Design review of the part built by this model. Coordinates are the model's own, in mm. A direction names the side the tool comes from. Coordinates: 2 decimals unless noted, no trailing zeros. Write each loop counter-clockwise with the first axis right and the second up, starting at its lowest first coordinate (ties: lowest second). Pieces come first, ordered by that corner, then holes.
Q1. Clearance check with flat-ended pins moving along their axes: pin 1 Ø1.5 at (x, y) = (6, 11) entering from +Z; pin 2 Ø1 at (x, y) = (9, -10.5) entering from -Z; pin 3 Ø10 at (x, y) = (6.5, 12) entering from +Z. State where each tip first meets the part, or that it passes through.
Q2. Add section D-D, the plane y = -15.5. Give the boundary of the cut face in (x, z), plus the area to 3 significant figures.
Q3. Add section A-A, the plane z = 0. Give the boundary of the cut face in (x, y), plus the area to 3 significant figures.
Q4. The part is to be moulded in two halves that separate along Z. For faces 4 (the face through (0.14, 7.509, -23.846)), 5 (the face through (-10, 0, 11)), 6 (the face through (-7, 0, 2.5)), say which applies: +Z half, -Z half, draft (parallel to the pull), parting line (faces both ways), or undercut.
Q5. Add section C-C, the plane x = 19. Give the boundary of the cut face in (y, z).
Q6. Machinability: for faces 1 (the face through (-10, 0, -11)), 2 (the face through (-7, 0, -2.5)), 3 (the face through (16.93, -4.88, 1.08)), which of the approach directions +Z, -Z, +X, -X, +Y, -Y give a long, thin tool a straight path to every point of the face, cutting with its end or side? Answer none if there is none.
Q7. Add section B-B, the plane y = 0. Give the boundary of the cut face in (x, z).
Q8. To check wall thickness, follow probe 1 along X at (y, z) = (-20, 14); probe 2 along Z at (x, y) = (-1, -2.5); probe 3 along Z at (x, y) = (14, 0). State the ranges of each line that lie inside material, in increasing order.
from build123d import *

# Parameters (mm, degrees)
SKETCH1_R           = 25
BOSS_EXTRUDE1_DEPTH = 10
SKETCH2_R           = 5
BOSS_EXTRUDE2_DEPTH = 12
CUT_EXTRUDE1_START  = -5
CUT_EXTRUDE1_DEPTH  = 5
SKETCH4_R           = 10
BOSS_EXTRUDE3_DEPTH = 2


with BuildPart() as part:
    # Sketch1 → Boss-Extrude1 (new, symmetric)
    with BuildSketch(Plane(origin=(0, 0, 0), x_dir=(0, 0, -1), z_dir=(1, 0, 0))):
        Circle(SKETCH1_R)
    extrude(amount=BOSS_EXTRUDE1_DEPTH, both=True)

    # Sketch2 → Boss-Extrude2 (add)
    with BuildSketch(Plane(origin=(10, 0, 0), x_dir=(0, 0, -1), z_dir=(1, 0, 0))):
        Circle(SKETCH2_R)
    extrude(amount=BOSS_EXTRUDE2_DEPTH)

    # Sketch3 → Cut-Extrude1 (cut)
    with BuildSketch(Plane.ZY.offset(10).offset(CUT_EXTRUDE1_START)):
        with BuildLine():
            Line((2.5, 24.874685928), (2.5, -24.874685928))
            ThreePointArc((2.5, -24.874685928), (0, -25), (-2.5, -24.874685928))
            Line((-2.5, -24.874685928), (-2.5, 24.874685928))
            ThreePointArc((-2.5, 24.874685928), (0, 25), (2.5, 24.874685928))
        make_face()
    extrude(amount=CUT_EXTRUDE1_DEPTH, mode=Mode.SUBTRACT)

    # Sketch4 → Boss-Extrude3 (add)
    with BuildSketch(Plane(origin=(10, 0, 0), x_dir=(0, 0, -1), z_dir=(1, 0, 0))):
        Circle(SKETCH4_R)
    extrude(amount=BOSS_EXTRUDE3_DEPTH)


solid = part.part
Here are the results:
1. pin 1: stops at z = 22.8
1. pin 2: stops at z = -22.91
1. pin 3: stops at z = 24
2. outline: (-10, -19.62) - (10, -19.62) - (10, 19.62) - (-10, 19.62) - (-10, 2.5) - (-5, 2.5) - (-5, -2.5) - (-10, -2.5) - close
2. area: 760 mm2
3. outline: (-5, -25) - (10, -25) - (10, -10) - (12, -10) - (12, -5) - (22, -5) - (22, 5) - (12, 5) - (12, 10) - (10, 10) - (10, 25) - (-5, 25) - close
3. area: 890 mm2
4. face 4: parting line
4. face 5: draft
4. face 6: undercut
5. outline: circle Ø10 at (0, 0)
6. face 1: +Z, -Z, -X, +Y, -Y
6. face 2: -X, +Y, -Y
6. face 3: +X
7. outline: (-10, -25) - (10, -25) - (10, -10) - (12, -10) - (12, -5) - (22, -5) - (22, 5) - (12, 5) - (12, 10) - (10, 10) - (10, 25) - (-10, 25) - (-10, 2.5) - (-5, 2.5) - (-5, -2.5) - (-10, -2.5) - close
8. probe 1: x = -10 to 10
8. probe 2: z = -24.87 to 24.87
8. probe 3: z = -5 to 5
